from build123d import *

# Parameters (mm, degrees)
BOSS_EXTRUDE1_OUTLINE_R = 0.25
BOSS_EXTRUDE1_DEPTH     = 0.4
BOSS_EXTRUDE2_DEPTH     = 1
BOSS_EXTRUDE3_START     = 0.8
BOSS_EXTRUDE3_DEPTH     = 0.2


# Read off the part's stored shape, not the designer's step: Boss-Extrude1
with BuildPart() as part:
    # Boss-Extrude1 outline → Boss-Extrude1 (new body)
    with BuildSketch(Plane.XY):
        with BuildLine():
            ThreePointArc((0.232880573, 11.939538652), (-0.004933085, 11.711410613), (-0.295707305, 11.556336146))
            Line((-0.295707305, 11.556336146), (-0.267193244, 11.23041893))
            Line((-0.267193244, 11.23041893), (-0.864910062, 11.178125485))
            Line((-0.864910062, 11.178125485), (-0.893424124, 11.5040427))
            ThreePointArc((-0.893424124, 11.5040427), (-1.206709229, 11.606268825), (-1.480523981, 11.789635178))
            ThreePointArc((-1.480523981, 11.789635178), (-1.381646187, 11.58978807), (-1.238910718, 11.418492212))
            ThreePointArc((-1.238910718, 11.418492212), (-1.124081641, 11.241613378), (-1.102444702, 11.031842833))
            ThreePointArc((-1.102444702, 11.031842833), (-0.830623384, 10.84424284), (-0.708470889, 10.537388877))
            Line((-0.708470889, 10.537388877), (-0.298379869, 5.850027068))
            ThreePointArc((-0.298379869, 5.850027068), (-0.406499279, 5.430691492), (-0.75404158, 5.172338089))
            ThreePointArc((-0.75404158, 5.172338089), (-1.129720091, 5.078868092), (-1.509480558, 5.003681847))
            ThreePointArc((-1.509480558, 5.003681847), (-1.666132979, 5.034974657), (-1.792562668, 5.132620725))
            Line((-1.792562668, 5.132620725), (-1.875378571, 5.387501866))
            ThreePointArc((-1.875378571, 5.387501866), (-1.925085173, 5.445700819), (-2.001385922, 5.451705818))
            Line((-2.001385922, 5.451705818), (-2.686146614, 5.229213582))
            ThreePointArc((-2.686146614, 5.229213582), (-2.744345567, 5.179506981), (-2.750350566, 5.103206231))
            Line((-2.750350566, 5.103206231), (-2.479687932, 4.270192298))
            Line((-2.479687932, 4.270192298), (-2.259859524, 4.046679542))
            Line((-2.259859524, 4.046679542), (-2.202796133, 4.065220562))
            Line((-2.202796133, 4.065220562), (-2.529237563, 5.069903979))
            Line((-2.529237563, 5.069903979), (-2.034688175, 5.230592816))
            Line((-2.034688175, 5.230592816), (-1.710220331, 4.231983473))
            ThreePointArc((-1.710220331, 4.231983473), (-0.998592576, 4.592140334), (-0.223827126, 4.40275838))
            ThreePointArc((-0.223827126, 4.40275838), (0.010695557, 4.334415883), (0.241228985, 4.415198467))
            ThreePointArc((0.241228985, 4.415198467), (1.395767253, 4.789072574), (2.533587129, 4.367045296))
            Line((2.533587129, 4.367045296), (3.111517477, 5.240202804))
            Line((3.111517477, 5.240202804), (3.555740915, 4.968344082))
            Line((3.555740915, 4.968344082), (2.879966638, 3.947360522))
            Line((2.879966638, 3.947360522), (2.929999788, 3.914244302))
            Line((2.929999788, 3.914244302), (3.214623401, 4.09061153))
            Line((3.214623401, 4.09061153), (3.779706708, 4.944359277))
            ThreePointArc((3.779706708, 4.944359277), (3.793941313, 5.021225846), (3.748517476, 5.084847921))
            Line((3.748517476, 5.084847921), (3.133596604, 5.46117116))
            ThreePointArc((3.133596604, 5.46117116), (3.059724383, 5.473499401), (2.998008671, 5.431069912))
            Line((2.998008671, 5.431069912), (2.974770776, 5.395961283))
            ThreePointArc((2.974770776, 5.395961283), (2.570340353, 5.081865355), (2.058285642, 5.077371822))
            ThreePointArc((2.058285642, 5.077371822), (1.543060021, 5.181767476), (1.017672926, 5.163759347))
            ThreePointArc((1.017672926, 5.163759347), (0.40272096, 5.32561867), (0.10009801, 5.884889365))
            Line((0.10009801, 5.884889365), (-0.30999301, 10.572251175))
            ThreePointArc((-0.30999301, 10.572251175), (-0.242980918, 10.895654894), (-0.007865573, 11.127606098))
            ThreePointArc((-0.007865573, 11.127606098), (-0.022983621, 11.337946973), (0.059386258, 11.53207848))
            ThreePointArc((0.059386258, 11.53207848), (0.170208041, 11.725557722), (0.232880573, 11.939538652))
        make_face()
        with Locations((0, 4.734272207)):
            Circle(BOSS_EXTRUDE1_OUTLINE_R, mode=Mode.SUBTRACT)
    extrude(amount=BOSS_EXTRUDE1_DEPTH)

    # Sketch1<8> → Boss-Extrude2 (add)
    with BuildSketch(Plane.XY):
        Polygon((-0.365402387, 10.918740425), (-0.321824516, 10.420643076), (-0.67049266, 10.390138566), (-0.714070532, 10.888235915), align=None)
    extrude(amount=BOSS_EXTRUDE2_DEPTH)

    # Sketch1<9> → Boss-Extrude3 (add)
    with BuildSketch(Plane.XY.offset(BOSS_EXTRUDE3_START)):
        Polygon((-0.624413009, 10.896079932), (-0.45505991, 10.910896408), (-0.54245757, 11.909856226), (-0.639965564, 12.049112073), (-0.711810668, 11.895039749), align=None)
    extrude(amount=BOSS_EXTRUDE3_DEPTH)


solid = part.part
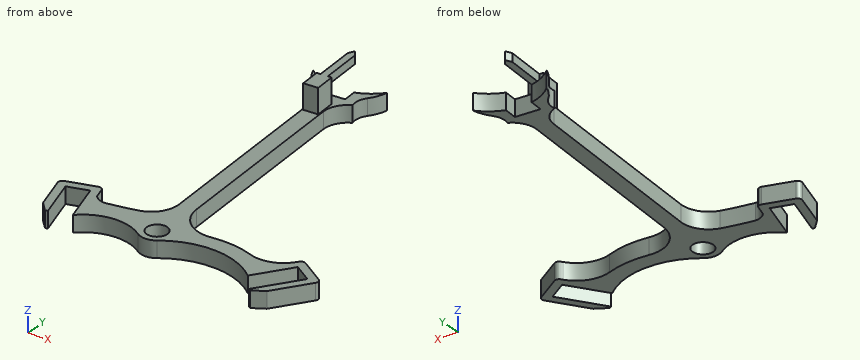
Here's how the part is built. I have some questions about the finished solid (model axes, mm). Give positions to 0.01 mm unless a question says otherwise; leave off trailing zeros. Loops run counter-clockwise (first coordinate to the right, second up) from the corner with the lowest first, then second, coordinate; pieces in that order, holes last. Notation, with made-up numbers: (23.5, -14.75) -> (46.5, -14.75) arc R29 cw to (46.5, 7.25) -> close; hole circle Ø8 at (75.5, 71.5). An arc over 180 degrees is marked (long way). Answer as a JSON object with one key per item and string values. Group by question number.
Item 1: Imagine slicing it at C-C on y = 10. Write out the boundary of the cut face in (x, z).
Item 2: Imagine slicing it at A-A on z = 0.9. Write out the boundary of the cut face in (x, y), then the cut area to 3 significant figures.
Item 3: I need wall thicknesses on L1, parallel to X at y = 5.75, z = 0.15; L2, parallel to X at y = 7.25, z = 0.1; L3, parallel to Y at x = 2, z = 0.2. Which ranges of each line are inside material? Lowest first, please.
Item 4: Will this pin go through, and if not, where does the flat tip stop? pin 1 (2 mm diameter, centred on x = -1, y = 5, fed in from +Z).
Item 5: Imagine slicing it at B-B on x = -1. Write out the boundary of the cut face in (y, z).
Answer list:
{
 "1": {"outline": "(-0.66, 0) -> (-0.26, 0) -> (-0.26, 0.4) -> (-0.66, 0.4) -> close"},
 "2": {"outline": "(-0.71, 10.89) -> (-0.67, 10.39) -> (-0.32, 10.42) -> (-0.37, 10.92) -> (-0.46, 10.91) -> (-0.54, 11.91) -> (-0.64, 12.05) -> (-0.71, 11.9) -> (-0.62, 10.9) -> close", "area": "0.358 mm2"},
 "3": {"L1": "x = -0.3 to 0.12", "L2": "x = -0.42 to -0.02", "L3": "y = 4.67 to 5.1"},
 "4": {"pin 1": "stops at z = 0.4"},
 "5": {"outline": "(4.59, 0) -> (5.11, 0) -> (5.11, 0.4) -> (4.59, 0.4) -> close; (10.99, 0) -> (11.53, 0) -> (11.53, 0.4) -> (10.99, 0.4) -> close"}
}
